Check sheet for the drawn part. Datum: minimum x, y, z corner. Units: mm. Give positions to 0.01 mm unless a question says otherwise; leave off trailing zeros. Order: outer loops, then holes, each group sorted by start corner. A loop starts at its lowest first (then second) coordinate and runs counter-clockwise, first axis right, second up.
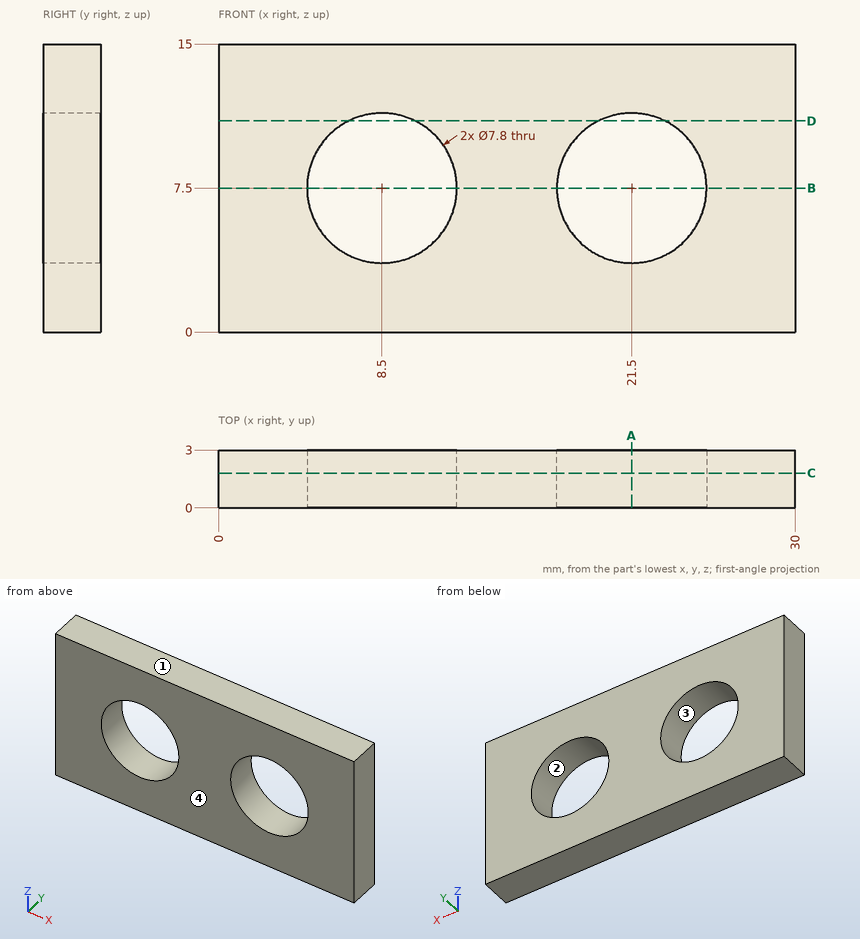
(1) Section check D-D, the plane z = 11. Enter the section's corners in (x, y), then the cut area to 3 significant figures.
Solved:
outline: (0, 0) - (6.78, 0) - (6.78, 3) - (0, 3) - close; (10.22, 0) - (19.78, 0) - (19.78, 3) - (10.22, 3) - close; (23.22, 0) - (30, 0) - (30, 3) - (23.22, 3) - close
area: 69.4 mm2
(2) Section check C-C, the plane y = 1.8. Enter the section's corners in (x, z), then the cut area to 3 significant figures.
Solved:
outline: (0, 0) - (30, 0) - (30, 15) - (0, 15) - close; hole circle Ø7.8 at (8.5, 7.5); hole circle Ø7.8 at (21.5, 7.5)
area: 354 mm2
(3) Release check for a two-part mould opening along Z. For the marked faces 1, 2, 3 and 4 record: pulls with the +Z half, pulls with the -Z half, needs draft (parallel to the pull), parting line crosses it, or undercut.
Solved:
face 1: pulls with the +Z half
face 2: undercut
face 3: undercut
face 4: needs draft
(4) Section check B-B, the plane z = 7.5. Enter the section's corners in (x, y).
Solved:
outline: (0, 0) - (4.6, 0) - (4.6, 3) - (0, 3) - close; (12.4, 0) - (17.6, 0) - (17.6, 3) - (12.4, 3) - close; (25.4, 0) - (30, 0) - (30, 3) - (25.4, 3) - close
(5) Scan lines: line 1 (Z direction, x = 8.5, y = 1.95); line 2 (X direction, y = 2.75, z = 5.5); line 3 (X direction, y = 2.15, z = 10). Record each from-to range of solid material in increasing order.
Solved:
line 1: z = 0 to 3.6, 11.4 to 15
line 2: x = 0 to 5.15, 11.85 to 18.15, 24.85 to 30
line 3: x = 0 to 5.51, 11.49 to 18.51, 24.49 to 30
(6) Section check A-A, the plane x = 21.5. Enter the section's corners in (y, z).
Solved:
outline: (0, 0) - (3, 0) - (3, 3.6) - (0, 3.6) - close; (0, 11.4) - (3, 11.4) - (3, 15) - (0, 15) - close
